```python
from build123d import *

# Parameters (mm, degrees)
BOSS_EXTRUDE1_DEPTH = 7
SKETCH3_R           = 4
BOSS_EXTRUDE2_DEPTH = 20
SKETCH4_R           = 4
BOSS_EXTRUDE3_DEPTH = 20


with BuildPart() as part:
    # Sketch2 → Boss-Extrude1 (new body)
    with BuildSketch(Plane.XY):
        with BuildLine():
            Line((0, 0), (147, 0))
            ThreePointArc((147, 0), (167, 20), (147, 40))
            Line((147, 40), (0, 40))
            ThreePointArc((0, 40), (-20, 20), (0, 0))
        make_face()
    extrude(amount=BOSS_EXTRUDE1_DEPTH)

    # Sketch3 → Boss-Extrude2 (add)
    with BuildSketch(Plane.XY.offset(7)):
        with Locations((147, 20)):
            Circle(SKETCH3_R)
    extrude(amount=BOSS_EXTRUDE2_DEPTH)

    # Sketch4 → Boss-Extrude3 (add)
    with BuildSketch(Plane.XY.offset(7)):
        with Locations((0, 20)):
            Circle(SKETCH4_R)
    extrude(amount=BOSS_EXTRUDE3_DEPTH)


solid = part.part
```
The model under review builds one solid part; all positions refer to its coordinate system, in mm. A direction names the side the tool comes from. Round coordinates to 2 decimals unless told otherwise and drop trailing zeros. Loops run counter-clockwise (first coordinate to the right, second up) from the corner with the lowest first, then second, coordinate; pieces in that order, holes last. Notation, with made-up numbers: M 5.25,-15.5 L 20.25,-15.5 A21 cw 20.25,15.5 Z; hole C -37,76.5 d1. An arc over 180 degrees is marked long. Answer as a JSON object with one key per item and string values.
(1) Take a section at D-D on y = 37. Give the boundary of the cut face in (x, z), and give its area (3 significant figures).
Resolved:
{"outline": "M -10.54,0 L 157.54,0 L 157.54,7 L -10.54,7 Z", "area": "1,180 mm²"}
(2) To check wall thickness, follow line 1 along X through (y, z) = (19.5, 18.75); line 2 along Z through (x, y) = (105.5, 37); line 3 along X through (y, z) = (23, 10.5). State the ranges of each line that lie inside material, in increasing order.
Resolved:
{"line 1": "-3.97 to 3.97, 143.03 to 150.97", "line 2": "0 to 7", "line 3": "-2.65 to 2.65, 144.35 to 149.65"}
(3) Take a section at C-C on x = 77.5. Give the boundary of the cut face in (y, z), and give its area (3 significant figures).
Resolved:
{"outline": "M 0,0 L 40,0 L 40,7 L 0,7 Z", "area": "280 mm²"}
(4) Take a section at B-B on y = 20. Give the boundary of the cut face in (x, z), and give its area (3 significant figures).
Resolved:
{"outline": "M -20,0 L 167,0 L 167,7 L 151,7 L 151,27 L 143,27 L 143,7 L 4,7 L 4,27 L -4,27 L -4,7 L -20,7 Z", "area": "1,630 mm²"}
(5) Draft analysis for pull direction X (two halves, no side actions). For faces 1 (the cylindrical face through (167, 20, 3)), 2 (the cylindrical face through (-0.521, 23.966, 16.86)), 3 (the flat face through (0, 20, 27)), state which applies: released by +X, released by -X, zero draft, split by the parting line, or undercut.
Resolved:
{"face 1": "released by +X", "face 2": "undercut", "face 3": "zero draft"}
(6) Tool access review of faces 4 (the cylindrical face through (150.815, 21.201, 16.86)), 5 (the flat face through (75, 40, 3)): name each direction out of +Z, -Z, +X, -X, +Y, -Y from which nothing blocks a thin tool from reaching the whole face with its end or side.
Resolved:
{"face 4": "+Z", "face 5": "+Z, -Z, +X, -X, +Y"}
(7) Clearance check with flat-ended pins moving along their axes: P1, Ø4, axis at y = 4.5, z = 3, coming from the +X side; P2, Ø3, axis at x = 113, y = 15.5, coming from the +Z side; P3, Ø1, axis at y = 31.5, z = 8, coming from the +X side; P4, Ø1.5, axis at y = 18.5, z = 11, coming from the -X side. State where each tip first meets the part, or that it passes through.
Resolved:
{"P1": "x = 161.76", "P2": "z = 7", "P3": "through", "P4": "x = -3.93"}
(8) Take a section at A-A on z = 9. Give the boundary of the cut face in (x, y), and give its area (3 significant figures).
Resolved:
{"outline": "C 0,20 d8; C 147,20 d8", "area": "101 mm²"}
